from build123d import *

# Parameters (mm, degrees)
SKETCH_1_R          = 5
EXTRUDE_1_DEPTH     = 108
CHAMFER_1_SIZE      = 0.5
CUT_EXTRUDE_START   = -3
SKETCH_2_R          = 5
SKETCH_2_R_2        = 4.8
CUT_EXTRUDE_1_DEPTH = 1.1


with BuildPart() as part:
    # 草图1 → 凸台-拉伸1 (new body)
    with BuildSketch(Plane(origin=(0, 0, 0), x_dir=(1, 0, 0), z_dir=(0, 1, 0))):
        with Locations(Location((0, 0, 0), (0, 0, 270))):
            Circle(SKETCH_1_R)
    extrude(amount=EXTRUDE_1_DEPTH)

    # 倒角1
    chamfer_1_edges = [part.edges().sort_by_distance(p)[0] for p in [
        (0, 0, -5),
        (0, 108, -5),
    ]]
    chamfer(chamfer_1_edges, length=CHAMFER_1_SIZE)

    # 草图2 → 切除-拉伸1 (cut)
    with BuildSketch(Plane(origin=(0, 108, 0), x_dir=(1, 0, 0), z_dir=(0, 1, 0)).offset(CUT_EXTRUDE_START)):
        with Locations(Location((0, 0, 0), (0, 0, 270))):
            Circle(SKETCH_2_R)
        with Locations(Location((0, 0, 0), (0, 0, 270))):
            Circle(SKETCH_2_R_2, mode=Mode.SUBTRACT)
    cut_extrude_1 = extrude(amount=CUT_EXTRUDE_1_DEPTH, mode=Mode.SUBTRACT)

    # 镜向1: 切除-拉伸1 across plane
    add(cut_extrude_1.mirror(Plane.ZX.offset(54)), mode=Mode.SUBTRACT)


solid = part.part
Check sheet for the modelled part. Datum: model origin and axes. Units: mm. A direction names the side the tool comes from. Give positions to 0.01 mm unless a question says otherwise; leave off trailing zeros. Write each loop counter-clockwise with the first axis right and the second up, starting at its lowest first coordinate (ties: lowest second). Pieces come first, ordered by that corner, then holes. Notation, with made-up numbers: (-8, 86.25) -> (35, 86.25) arc R10 cw to (35, 98.25) -> close; hole circle Ø3 at (-12.5, -17.75). An arc over 180 degrees is marked (long way). One line per item, written item: value. Start each with the question number.
Item 1: Material ranges on probe 1 along Z at (x, y) = (-0.25, 81); probe 2 along Z at (x, y) = (-0.75, 20.5); probe 3 along X at (y, z) = (24.5, 2), recorded low to high. Write a range as from..to.
Item 2: Tool access check on faces 4 (the cylindrical face through (4.05, 105.54, 2.58)), 5 (the flat face through (0, 108, 0)). Record the directions out of +Z, -Z, +X, -X, +Y, -Y that give a thin tool (end or side, any length) a straight path to the whole face; none if there is none.
Item 3: Section check A-A on y = 17.5. Record the cut outline in (x, z).
Item 4: Draft check along Y on faces 1 (the cylindrical face through (4.05, 2.46, 2.58)), 2 (the flat face through (0, 0, 0)), 3 (the cylindrical face through (-4.88, 1.19, -1.08)). Enter one of: +Y half, -Y half, draft (parallel to the pull), parting line (faces both ways), or undercut.
Item 5: Gauge pin test, flat ends, axial feed: pin 1 (2 mm diameter, centred on y = 96, z = -2.5, fed in from +X); pin 2 (6 mm diameter, centred on x = -3, y = 40.5, fed in from +Z); pin 3 (6 mm diameter, centred on y = 52, z = -3.5, fed in from -X). Record the tip position at first contact, or that the pin passes through.
Results list:
1. probe 1: -4.99..4.99
1. probe 2: -4.94..4.94
1. probe 3: -4.58..4.58
2. face 4: none
2. face 5: +Z, -Z, +X, -X, +Y
3. outline: circle Ø10 at (0, 0)
4. face 1: undercut
4. face 2: -Y half
4. face 3: draft
5. pin 1: x = 4.77
5. pin 2: z = 5
5. pin 3: x = -4.97
